```python
from build123d import *

# Parameters (mm, degrees)
SKETCH1_R            = 38.1
BOSS_EXTRUDE1_DEPTH  = 19.05
FILLET1_R            = 12.7
SKETCH2_R            = 41.275
BOSS_EXTRUDE2_DEPTH  = 3.175
SHELL2_T             = -2.54
FILLET2_R            = 2.54
SKETCH27_W           = 5.08
SKETCH27_H           = 5.08
BOSS_EXTRUDE12_DEPTH = 3.175
FILLET3_R            = 1.27
SKETCH28_R           = 38.735
SKETCH28_R_2         = 35.56
BOSS_EXTRUDE16_DEPTH = 0.635
SKETCH31_R           = 6
SKETCH31_R_2         = 4.5
BOSS_EXTRUDE17_DEPTH = 19.685
FILLET4_R            = 8.89
SKETCH32_R           = 6
BOSS_EXTRUDE18_DEPTH = 1.27
FILLET5_R            = 2.54


with BuildPart() as part:
    # Sketch1 → Boss-Extrude1 (new body)
    with BuildSketch(Plane(origin=(0, 0, 0), x_dir=(1, 0, 0), z_dir=(0, 1, 0))):
        with Locations(Location((0, 0, 0), (0, 0, 90))):
            Circle(SKETCH1_R)
    extrude(amount=BOSS_EXTRUDE1_DEPTH)

    # Fillet1
    fillet1_edges = [part.edges().sort_by_distance(p)[0] for p in [
        (0, 19.05, 38.1),
    ]]
    fillet(fillet1_edges, radius=FILLET1_R)

    # Sketch2 → Boss-Extrude2 (add)
    with BuildSketch(Plane.XZ):
        with Locations(Location((0, 0, 0), (0, 0, 270))):
            Circle(SKETCH2_R)
    extrude(amount=BOSS_EXTRUDE2_DEPTH)

    # Shell2
    shell2_openings = [part.faces().sort_by_distance(p)[0] for p in [
        (0, -3.175, 0),
    ]]
    offset(amount=SHELL2_T, openings=shell2_openings, kind=Kind.INTERSECTION)

    # Fillet2
    fillet2_edges = [part.edges().sort_by_distance(p)[0] for p in [
        (0, 0, 38.1),
    ]]
    fillet(fillet2_edges, radius=FILLET2_R)

    # Sketch27 → Boss-Extrude12 (add)
    with BuildSketch(Plane.XZ.offset(3.175)):
        with Locations((-41.275, 0)):
            Rectangle(SKETCH27_W, SKETCH27_H)
        with Locations((0, 41.275)):
            Rectangle(SKETCH27_W, SKETCH27_H)
        with Locations((41.275, 0)):
            Rectangle(SKETCH27_W, SKETCH27_H)
        with Locations((0, -41.275)):
            Rectangle(SKETCH27_W, SKETCH27_H)
    extrude(amount=-BOSS_EXTRUDE12_DEPTH)

    # Fillet3
    fillet3_edges = [part.edges().sort_by_distance(p)[0] for p in [
        (-2.54, -1.5875, 41.196772022),
        (2.54, -1.5875, 41.196772022),
        (41.196772022, -1.5875, 2.54),
        (41.196772022, -1.5875, -2.54),
        (2.54, -1.5875, -41.196772022),
        (-2.54, -1.5875, -41.196772022),
        (-41.196772022, -1.5875, -2.54),
        (-41.196772022, -1.5875, 2.54),
    ]]
    fillet(fillet3_edges, radius=FILLET3_R)

    # Sketch28 → Boss-Extrude16 (add)
    with BuildSketch(Plane.XZ.offset(2.54)):
        Circle(SKETCH28_R)
        with Locations(Location((0, 0, 0), (0, 0, 270))):
            Circle(SKETCH28_R_2, mode=Mode.SUBTRACT)
    extrude(amount=BOSS_EXTRUDE16_DEPTH)

    # Sketch31 → Boss-Extrude17 (add)
    with BuildSketch(Plane.XZ.offset(-16.51)):
        with Locations(Location((0, 0, 0), (0, 0, 90))):
            Circle(SKETCH31_R)
        with Locations(Location((0, 0, 0), (0, 0, 90))):
            Circle(SKETCH31_R_2, mode=Mode.SUBTRACT)
    extrude(amount=BOSS_EXTRUDE17_DEPTH)

    # Fillet4
    fillet4_edges = [part.edges().sort_by_distance(p)[0] for p in [
        (0, 16.51, -6),
    ]]
    fillet(fillet4_edges, radius=FILLET4_R)

    # Sketch32 → Boss-Extrude18 (add)
    with BuildSketch(Plane.XZ.offset(3.175)):
        with Locations(Location((0, 0, 0), (0, 0, 90))):
            Circle(SKETCH32_R)
    extrude(amount=-BOSS_EXTRUDE18_DEPTH)

    # Fillet5
    fillet5_edges = [part.edges().sort_by_distance(p)[0] for p in [
        (0, -1.905, -4.5),
    ]]
    fillet(fillet5_edges, radius=FILLET5_R)


solid = part.part
```
The listing builds one solid part. Answer for the finished solid, in the listing's coordinates (mm). A direction names the side the tool comes from. Coordinates: 2 decimals unless noted, no trailing zeros. Order: outer loops, then holes, each group sorted by start corner. A loop starts at its lowest first (then second) coordinate and runs counter-clockwise, first axis right, second up. Notation, with made-up numbers: M -8,-12.75 L 28,-12.75 A14 ccw 28,5.25 Z; hole C 40.25,30 d3. An arc over 180 degrees is marked long. Answer as a JSON object with one key per item and string values. Group by question number.
1. Section A-A on y = 3.75 is taken. Write down the section's boundary in (x, z), then the cut area to 3 significant figures.
2. Section B-B on y = 9 is taken. Write down the section's boundary in (x, z), then the cut area to 3 significant figures.
3. Straight lines are drawn through the part: line 1 (X direction, y = 3.25, z = 0); line 2 (X direction, y = 14.25, z = -4); line 3 (X direction, y = -1.5, z = 3.5). For each, find the intervals that lie inside material, in ascending order.
4. A tool of negligible diameter and unlimited length cuts with its end or side. For faces 4 (the cylindrical face through (-1.352, 8.684, 4.292)), 5 (the flat face through (0, -2, 43.815)), 6 (the flat face through (39, 0, -13)), 7 (the cylindrical face through (-1.802, 2.298, 5.723)), from which of +Z, -Z, +X, -X, +Y, -Y can it reach the whole face along a straight path? Write none if from no direction.
5. Flat-ended cylindrical pins translate along their axes: P1, Ø0.7, axis at x = 43, y = -1.5, coming from the -Z side; P2, Ø0.7, axis at y = -1.5, z = 43, coming from the +X side; P3, Ø10, axis at x = -10, y = 6, coming from the +Z side. Find the tip coordinate at first contact, or state that the pin passes through.
6. Determine the mould class of faces 1 (the cylindrical face through (-28.9, -1.57, 29.47)), 2 (the flat face through (-6.7, -3.175, -35.5)), 3 (the cylindrical face through (-34.714, 1.654, 7.709)) for opening direction Z: released by +Z, released by -Z, zero draft, split by the parting line, or undercut.
Values follow:
{
 "1": {"outline": "C 0,0 d76.2; C 0,0 d12; hole C 0,0 d71.12; hole C 0,0 d9", "area": "637 mm2"},
 "2": {"outline": "C 0,0 d75.64; C 0,0 d12.22; hole C 0,0 d70.42; hole C 0,0 d9", "area": "653 mm2"},
 "3": {"line 1": "-38.1 to -35.56, -6 to -4.5, 4.5 to 6, 35.56 to 38.1", "line 2": "-35.12 to -31.54, -8.03 to -2.06, 2.06 to 8.03, 31.54 to 35.12", "line 3": "-41.14 to -35.39, -4.87 to 4.87, 35.39 to 41.14"},
 "4": {"face 4": "none", "face 5": "+Z, +X, -X, +Y, -Y", "face 6": "+Y", "face 7": "-Y"},
 "5": {"P1": "z = -2.54", "P2": "x = 2.54", "P3": "z = 37.77"},
 "6": {"face 1": "released by +Z", "face 2": "zero draft", "face 3": "undercut"}
}
